Geometry check sheet. Reference: the model listing, model coordinates, mm. Face numbers are marked on the shaded views. A direction names the side the tool comes from. Give positions to 0.01 mm unless a question says otherwise; leave off trailing zeros. Loops run counter-clockwise (first coordinate to the right, second up) from the corner with the lowest first, then second, coordinate; pieces in that order, holes last.
```python
from build123d import *

# Parameters (mm, degrees)
F1_DEPTH = 60
F3_DEPTH = 120.001
F5_DEPTH = 20.001


with BuildPart() as f1:
    # F0 (on Front) → F1 (new body)
    with BuildSketch(Plane.XZ):
        with BuildLine():
            Line((-80, -10), (-80, -30))
            Line((-80, -30), (80, -30))
            Line((80, -30), (80, -10))
            Line((80, -10), (40, -10))
            Line((40, -10), (40, 30))
            Line((40, 30), (30, 30))
            ThreePointArc((30, 30), (0, 0), (-30, 30))
            Line((-30, 30), (-40, 30))
            Line((-40, 30), (-40, -10))
            Line((-40, -10), (-80, -10))
        make_face()
    extrude(amount=F1_DEPTH)

    # F2 (on face) → F3 (cut, through all)
    with BuildSketch(Plane.YZ.offset(40)):
        with BuildLine():
            ThreePointArc((-30, 6.8799550533), (-24.3431457505, 9.2231008038), (-22, 14.8799550533))
            ThreePointArc((-22, 14.8799550533), (-35.6568542495, 20.5368093028), (-30, 6.8799550533))
        make_face()
    extrude(amount=-F3_DEPTH, mode=Mode.SUBTRACT)

    # F4 (on face) → F5 (cut, through all)
    with BuildSketch(Plane.XY.offset(-10)):
        with BuildLine():
            ThreePointArc((59, -45), (60.7573593129, -49.2426406871), (65, -51))
            Line((65, -51), (65, -45))
            Line((65, -45), (59, -45))
        make_face()
        with BuildLine():
            Line((65, -45), (65, -51))
            ThreePointArc((65, -51), (69.2426406871, -49.2426406871), (71, -45))
            Line((71, -45), (65, -45))
        make_face()
        with BuildLine():
            ThreePointArc((-71, -45), (-69.2426406871, -49.2426406871), (-65, -51))
            Line((-65, -51), (-65, -45))
            Line((-65, -45), (-71, -45))
        make_face()
        with BuildLine():
            Line((-65, -45), (-65, -51))
            ThreePointArc((-65, -51), (-60.7573593129, -49.2426406871), (-59, -45))
            Line((-59, -45), (-65, -45))
        make_face()
        with BuildLine():
            Line((-71, -45), (-65, -45))
            Line((-65, -45), (-65, -39))
            ThreePointArc((-65, -39), (-69.2426406871, -40.7573593129), (-71, -45))
        make_face()
        with BuildLine():
            Line((-65, -39), (-65, -45))
            Line((-65, -45), (-59, -45))
            ThreePointArc((-59, -45), (-60.7573593129, -40.7573593129), (-65, -39))
        make_face()
        with BuildLine():
            Line((-71, -15), (-71, -45))
            ThreePointArc((-71, -45), (-69.2426406871, -40.7573593129), (-65, -39))
            ThreePointArc((-65, -39), (-60.7573593129, -40.7573593129), (-59, -45))
            Line((-59, -45), (-59, -15))
            ThreePointArc((-59, -15), (-65, -21), (-71, -15))
        make_face()
        with BuildLine():
            Line((59, -45), (65, -45))
            Line((65, -45), (65, -39))
            ThreePointArc((65, -39), (60.7573593129, -40.7573593129), (59, -45))
        make_face()
        with BuildLine():
            Line((65, -39), (65, -45))
            Line((65, -45), (71, -45))
            ThreePointArc((71, -45), (69.2426406871, -40.7573593129), (65, -39))
        make_face()
        with BuildLine():
            Line((59, -15), (59, -45))
            ThreePointArc((59, -45), (60.7573593129, -40.7573593129), (65, -39))
            ThreePointArc((65, -39), (69.2426406871, -40.7573593129), (71, -45))
            Line((71, -45), (71, -15))
            ThreePointArc((71, -15), (65, -21), (59, -15))
        make_face()
        with BuildLine():
            ThreePointArc((-59, -15), (-65, -9), (-71, -15))
            Line((-71, -15), (-59, -15))
        make_face()
        with BuildLine():
            Line((-59, -15), (-71, -15))
            ThreePointArc((-71, -15), (-65, -21), (-59, -15))
        make_face()
        with BuildLine():
            ThreePointArc((71, -15), (65, -9), (59, -15))
            Line((59, -15), (71, -15))
        make_face()
        with BuildLine():
            Line((71, -15), (59, -15))
            ThreePointArc((59, -15), (65, -21), (71, -15))
        make_face()
    extrude(amount=-F5_DEPTH, mode=Mode.SUBTRACT)


solid = f1.part
```
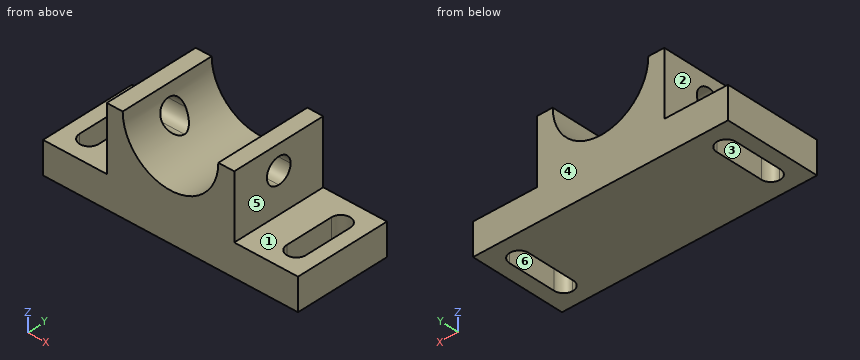
1) Mould release check, pull along Y, two halves, no side actions. Record for the marked faces 4, 5 and 6: +Y half, -Y half, draft (parallel to the pull), parting line (faces both ways), or undercut.
2) Sectioned sample at B-B on z = 11.5. Enter the section's corners in (x, y).
3) Sectioned sample at D-D on x = -22. Enter the section's corners in (y, z).
4) Sectioned sample at C-C on x = 68. Enter the section's corners in (y, z), plus the area to 3 significant figures.
5) Depth check by flat-ended pin: P1, Ø5, axis at y = -24, z = 6, coming from the -X side; P2, Ø6, axis at y = -39, z = 18, coming from the +X side; P3, Ø20, axis at x = -64, y = -22.5, coming from the +Z side. Enter the tip coordinate at first touch or a pass-through.
6) Scan lines: line 1 along X through (y, z) = (-43, -10.5); line 2 along Z through (x, y) = (0.5, -54); line 3 along Z through (x, y) = (-34, -30). Record each from-to range of solid material in increasing order.
7) Tool access check on the marked faces 1, 2 and 3. Record the directions out of +Z, -Z, +X, -X, +Y, -Y that give a thin tool (end or side, any length) a straight path to the whole face; none if there is none.
8) Sectioned sample at A-A on y = -39.5. Enter the section's corners in (x, z), plus the area to 3 significant figures.
Determined:
1. face 4: +Y half
1. face 5: draft
1. face 6: undercut
2. outline: (-40, -60) - (-23.62, -60) - (-23.62, -37.25) - (-40, -37.25) - close; (-40, -22.75) - (-23.62, -22.75) - (-23.62, 0) - (-40, 0) - close; (23.62, -60) - (40, -60) - (40, -37.25) - (23.62, -37.25) - close; (23.62, -22.75) - (40, -22.75) - (40, 0) - (23.62, 0) - close
3. outline: (-60, -30) - (0, -30) - (0, 9.6) - (-23.99, 9.6) arc R8 cw to (-36.01, 9.6) - (-60, 9.6) - close
4. outline: (-60, -30) - (-50.2, -30) - (-50.2, -10) - (-60, -10) - close; (-9.8, -30) - (0, -30) - (0, -10) - (-9.8, -10) - close
4. area: 392 mm2
5. P1: stops at x = -40
5. P2: stops at x = 40
5. P3: stops at z = -10
6. line 1: x = -80 to -71, -59 to 59, 71 to 80
6. line 2: z = -30 to 0
6. line 3: z = -30 to 6.88, 22.88 to 30
7. face 1: +Z, +X, +Y, -Y
7. face 2: +Z, -X, +Y, -Y
7. face 3: +Z, -Z
8. outline: (-80, -30) - (-71, -30) - (-71, -10) - (-80, -10) - close; (-59, -30) - (59, -30) - (59, -10) - (40, -10) - (40, 30) - (30, 30) arc R30 cw to (-30, 30) - (-40, 30) - (-40, -10) - (-59, -10) - close; (71, -30) - (80, -30) - (80, -10) - (71, -10) - close
8. area: 4,510 mm2
